Read the model definition and answer for the solid it produces. Units are mm, in the model's axes. Coordinates: 2 decimals unless noted, no trailing zeros. Write each loop counter-clockwise with the first axis right and the second up, starting at its lowest first coordinate (ties: lowest second). Pieces come first, ordered by that corner, then holes. Notation, with made-up numbers: (28.25, 17) -> (44.25, 17) arc R31 ccw to (44.25, 56) -> close; hole circle Ø3 at (2, 8). An arc over 180 degrees is marked (long way). Use CSV: the item, a comma, the result in double quotes.
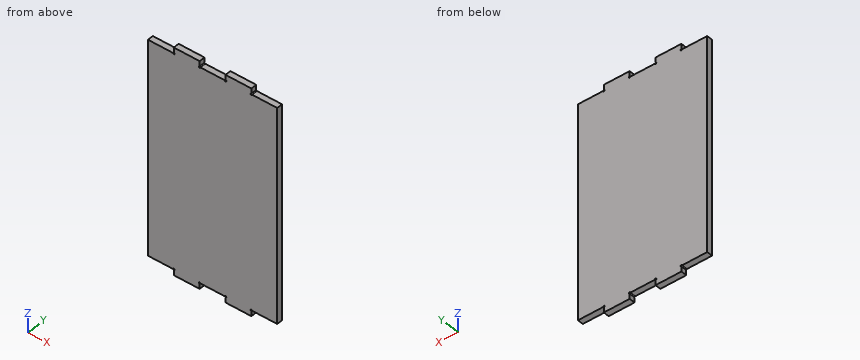
Autodesk Inventor part; units mm, degrees
ref_plane "YZ Plane" through (0, 0, 0) normal (1, 0, 0) x (0, 1, 0)
ref_plane "XZ Plane" through (0, 0, 0) normal (0, 1, 0) x (-1, 0, 0)
ref_plane "XY Plane" through (0, 0, 0) normal (0, 0, 1) x (1, 0, 0)
sketch "Sketch1" plane through (0, 0, 0) normal (0, 1, 0) x (-1, 0, 0)
  line L0 (400, 0) -> (400, -664)
  line L1 (0, -664) -> (0, 0)
  line L2 (320, 2.5) -> (320, 18)
  line L3 (80, 2.5) -> (80, 18)
  line L4 (320, 18) -> (240, 18)
  line L5 (160, 18) -> (80, 18)
  line L6 (322.5, 0) -> (400, 0)
  line L7 (0, 0) -> (77.5, 0)
  line L8 (162.5, 0) -> (237.5, 0)
  arc A0 (320, 2.5) -> (322.5, 0) centre (320, 0) ccw
  arc A1 (237.5, 0) -> (240, 2.5) centre (240, 0) ccw
  arc A2 (160, 2.5) -> (162.5, 0) centre (160, 0) ccw
  arc A3 (77.5, 0) -> (80, 2.5) centre (80, 0) ccw
  line L9 (240, 18) -> (240, 2.5)
  line L10 (160, 18) -> (160, 2.5)
  line L11 (320, -666.5) -> (320, -682)
  line L12 (80, -666.5) -> (80, -682)
  line L13 (320, -682) -> (240, -682)
  line L14 (160, -682) -> (80, -682)
  line L15 (322.5, -664) -> (400, -664)
  line L16 (0, -664) -> (77.5, -664)
  line L17 (162.5, -664) -> (237.5, -664)
  arc A4 (322.5, -664) -> (320, -666.5) centre (320, -664) ccw
  arc A5 (240, -666.5) -> (237.5, -664) centre (240, -664) ccw
  arc A6 (162.5, -664) -> (160, -666.5) centre (160, -664) ccw
  arc A7 (80, -666.5) -> (77.5, -664) centre (80, -664) ccw
  line L18 (240, -682) -> (240, -666.5)
  line L19 (160, -682) -> (160, -666.5)
  dimension "d4" = 80
  dimension "d13" = 18
  dimension "d20" = 5
  dimension "d21" = 5
  dimension "d22" = 5
  dimension "d23" = 5
  dimension "d28" = 80
  dimension "d29" = 18
  dimension "d30" = 80
  dimension "d31" = 18
  dimension "d33" = 80
  dimension "d34" = 18
  dimension "d36" = 18
  dimension "d37" = 664
extrude "Extrusion1" add sketch "Sketch1" along normal blind 18
properties part number "repisaa"
1. Each of these flat-tipped pins is pushed along its axis until it touches: pin 1 Ø4.5 at (y, z) = (12.5, 9.5) entering from -X; pin 2 Ø6.5 at (x, z) = (-320, 0) entering from +Y; pin 3 Ø9 at (x, y) = (-211.5, 9.5) entering from +Z; pin 4 Ø5.5 at (x, y) = (-199.5, 12.5) entering from -Z. Where does it stop, or does it pass through?
Solutions:
pin 1,"stops at x = -320"
pin 2,"stops at y = 18"
pin 3,"stops at z = 0"
pin 4,"stops at z = -664"
2. Find the intervals of material crossed by line 1 along Z through (x, y) = (-206.5, 8.25), in increasing order.
Solutions:
line 1,"z = -664 to 0"
3. A cutting plane is placed at A-A (y = 5). Give the vertices of the cut face in (x, z), and give its area (3 significant figures).
Solutions:
outline,"(-400, -664) -> (-322.5, -664) arc R2.5 cw (long way) to (-320, -666.5) -> (-320, -682) -> (-240, -682) -> (-240, -666.5) arc R2.5 cw (long way) to (-237.5, -664) -> (-162.5, -664) arc R2.5 cw (long way) to (-160, -666.5) -> (-160, -682) -> (-80, -682) -> (-80, -666.5) arc R2.5 cw (long way) to (-77.5, -664) -> (0, -664) -> (0, 0) -> (-77.5, 0) arc R2.5 cw (long way) to (-80, 2.5) -> (-80, 18) -> (-160, 18) -> (-160, 2.5) arc R2.5 cw (long way) to (-162.5, 0) -> (-237.5, 0) arc R2.5 cw (long way) to (-240, 2.5) -> (-240, 18) -> (-320, 18) -> (-320, 2.5) arc R2.5 cw (long way) to (-322.5, 0) -> (-400, 0) -> close"
area,"271,000 mm^2"
